Verification items for the finished model (mm, model axes). Face numbers are marked on the shaded views. A direction names the side the tool comes from. Round coordinates to 2 decimals unless told otherwise and drop trailing zeros. Order: outer loops, then holes, each group sorted by start corner. A loop starts at its lowest first (then second) coordinate and runs counter-clockwise, first axis right, second up. Notation, with made-up numbers: M 48.25,88 L 70.25,88 A27 cw 70.25,113 Z; hole C 1,12.5 d10. An arc over 180 degrees is marked long. One line per item, written item: value. Start each with the question number.
from build123d import *

# Parameters (mm, degrees)
BOSS_EXTRUDE2_START = -20.240625
BOSS_EXTRUDE2_DEPTH = 4.365625
SKETCH16_OUTSIDE_W  = 153.074
SKETCH16_OUTSIDE_H  = 154.794
SKETCH16_OUTSIDE_R  = 5.55625
CUT_EXTRUDE7_DEPTH  = 38.099499124
CUT_EXTRUDE7_DRAFT  = -60
FILLET1_R           = 0.762


with BuildPart() as part:
    # Sketch6 → Revolve1 (revolve)
    with BuildSketch(Plane.XY, mode=Mode.PRIVATE) as revolve1_sk:
        Polygon((9.525, 2.143125), (-3.357695036, 2.143125), (-5.2832, 2.6590625), (-15.875, 2.6590625), (-15.875, 5.55625), (-20.240625, 5.55625), (-20.240625, 0), (15.875, 0), (13.663446892, 1.295930736), align=None)
    revolve(revolve1_sk.sketch.rotate(Axis((-20.240625, 0, 0), (1, 0, 0)), 180), axis=Axis((-20.240625, 0, 0), (1, 0, 0)))

    # Sketch15 → Boss-Extrude2 (add)
    with BuildSketch(Plane(origin=(0, 0, 0), x_dir=(0, 0, -1), z_dir=(1, 0, 0)).offset(BOSS_EXTRUDE2_START)):
        Polygon((0, 6.415804866), (-5.55625, 3.207902433), (-5.55625, -3.207902433), (0, -6.415804866), (5.55625, -3.207902433), (5.55625, 3.207902433), align=None)
    extrude(amount=BOSS_EXTRUDE2_DEPTH)


with BuildPart() as cut_extrude7_tool:
    # Sketch16 outside → Cut-Extrude7 (with draft: the straight prism first)
    with BuildSketch(Plane.ZY.offset(20.240625)):
        Rectangle(SKETCH16_OUTSIDE_W, SKETCH16_OUTSIDE_H)
        Circle(SKETCH16_OUTSIDE_R, mode=Mode.SUBTRACT)
    extrude(amount=-CUT_EXTRUDE7_DEPTH)
    # Cut-Extrude7: the draft: its side faces are tilted about the plane it starts from
    cut_extrude7_sides = [cut_extrude7_tool.faces().sort_by_distance(p)[0] for p in [
        (-1.190875438, -77.397, 0),
        (-1.190875438, 0, 76.537),
        (-1.190875438, 77.397, 0),
        (-1.190875438, 0, -76.537),
        (-1.190875438, 0, -5.55625),
    ]]
    draft(cut_extrude7_sides, Plane.ZY.offset(20.240625), CUT_EXTRUDE7_DRAFT)


with BuildPart() as part_1:
    add(part.part)

    # Cut-Extrude7: cut by cut_extrude7_tool
    add(cut_extrude7_tool.part, mode=Mode.SUBTRACT)

    # Fillet1
    fillet1_edges = [part_1.edges().sort_by_distance(p)[0] for p in [
        (-15.875, 2.6590625, 0),
    ]]
    fillet(fillet1_edges, radius=FILLET1_R)


solid = part_1.part
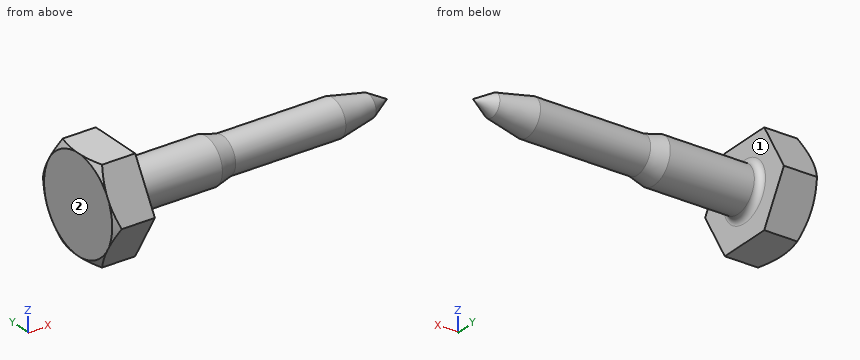
1. Depth check by flat-ended pin: pin 1 (3 mm diameter, centred on y = -2, z = 1.5, fed in from +X); pin 2 (6 mm diameter, centred on x = -9, y = 4.5, fed in from -Z). Enter the tip coordinate at first touch or a pass-through.
2. Section check C-C (x = 11). Record the cut outline in (y, z), and give its area (3 significant figures).
3. Scan lines: line 1 along X through (y, z) = (3.25, 2) (3 decimals); line 2 along Y through (x, z) = (1.5, 0.5); line 3 along X through (y, z) = (2, -2). Record each from-to range of solid material in increasing order.
4. Tool access check on the marked faces 1 and 2. Record the directions out of +Z, -Z, +X, -X, +Y, -Y that give a thin tool (end or side, any length) a straight path to the whole face; none if there is none.
5. Section check B-B (x = 4). Record the cut outline in (y, z), and give its area (3 significant figures).
6. Section check A-A (x = -18). Record the cut outline in (y, z).
Geometry check:
1. pin 1: stops at x = 14.17
1. pin 2: stops at z = -2.2
2. outline: C 0,0 d3.68
2. area: 10.6 mm²
3. line 1: x = -20.241 to -15.875
3. line 2: y = -2.08 to 2.08
3. line 3: x = -20.24 to -15.59
4. face 1: +X
4. face 2: +Z, -Z, -X, +Y, -Y
5. outline: C 0,0 d4.29
5. area: 14.4 mm²
6. outline: M -6.42,0 L -3.21,-5.56 L 3.21,-5.56 L 6.42,0 L 3.21,5.56 L -3.21,5.56 Z
